Could you check a few things on this model? Use its own coordinates, in mm. Give positions to 0.01 mm unless a question says otherwise; leave off trailing zeros. Write each loop counter-clockwise with the first axis right and the second up, starting at its lowest first coordinate (ties: lowest second). Pieces come first, ordered by that corner, then holes. Notation, with made-up numbers: (9, 60.5) - (36, 60.5) arc R16 ccw to (36, 65.5) - close; hole circle Ø9 at (70.5, 75). An arc over 180 degrees is marked (long way). Write item = value, one per line.
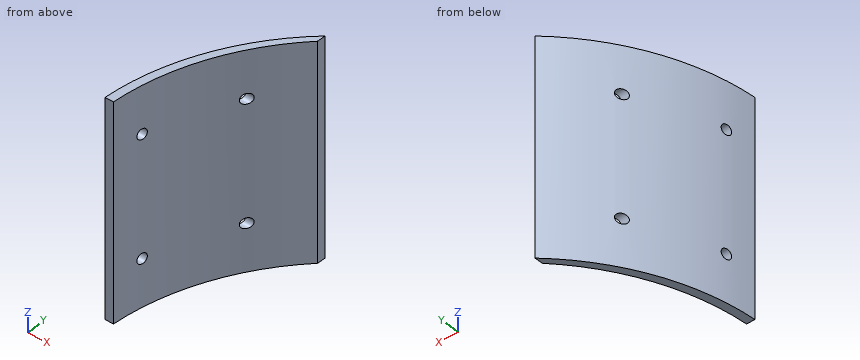
Autodesk Inventor part; units mm, degrees
ref_plane "YZ Plane" through (0, 0, 0) normal (1, 0, 0) x (0, 1, 0)
ref_plane "XZ Plane" through (0, 0, 0) normal (0, 1, 0) x (-1, 0, 0)
ref_plane "XY Plane" through (0, 0, 0) normal (0, 0, 1) x (1, 0, 0)
sketch "Sketch1" plane through (0, 0, 0) normal (0, 0, 1) x (1, 0, 0)
  arc A0 (45, 98) -> (0, 0) centre (139.9137, -4.9145) ccw
  line L0 (45, 98) -> (45, 93)
  line L1 (0, 0) -> (5, 0)
  arc A1 (45, 93) -> (5, 0) centre (144.908, -5.0734) ccw
  dimension "d0" = 140
  dimension "d1" = 98
  dimension "d3" = 45
  dimension "d4" = 5
  dimension "d5" = 5
  dimension "d6" = 140
extrude "Extrusion1" add sketch "Sketch1" along normal blind 125
sketch "Sketch2" plane through (0, 0, 0) normal (1, 0, 0) x (0, 1, 0)
  circle A0 centre (67.5, 27.5) radius 3
  circle A1 centre (17.5, 27.5) radius 3
  line L0 (98, 0) -> (98, 125)
  circle A2 centre (67.5, 97.5) radius 3
  circle A3 centre (17.5, 97.5) radius 3
  point P0 (0, 0)
  dimension "d9" = 6
  dimension "d10" = 6
  dimension "d11" = 27.5
  dimension "d12" = 50
  dimension "d13" = 30.5
  dimension "d14" = 6
  dimension "d15" = 6
  dimension "d16" = 70
extrude "Extrusion2" cut sketch "Sketch2" along normal through all
properties part number "SJ009" material "ABS Plastic"
1. If we section it at B-B, the plane z = 97.5: Please give me the cut outline in (x, y), and give its area (3 significant figures).
Filled sheet:
outline = (0, 0) - (5, 0) arc R140 cw to (6.28, 14.5) - (1.27, 14.5) arc R140 ccw to start; (2.24, 20.5) - (7.26, 20.5) arc R140 cw to (23.42, 64.5) - (18.33, 64.5) arc R140 ccw to start; (21.96, 70.5) - (27.06, 70.5) arc R140 cw to (45, 93) - (45, 98) arc R140 ccw to start
area = 423 mm2
2. If we section it at A-A, the plane y = 17: Please give me the cut outline in (x, z).
Filled sheet:
outline = (1.64, 0) - (6.66, 0) - (6.66, 24.54) - (1.64, 24.54) - close; (1.64, 30.46) - (6.66, 30.46) - (6.66, 94.54) - (1.64, 94.54) - close; (1.64, 100.46) - (6.66, 100.46) - (6.66, 125) - (1.64, 125) - close
3. I need wall thicknesses on line 1 (Z direction, x = 2.5, y = 17.5); line 2 (Y direction, x = 23, z = 97); line 3 (X direction, y = 12.5, z = 118). Which ranges of each line are inside material? Lowest first, please.
Filled sheet:
line_1 = 0 to 24.5, 30.5 to 94.5, 100.5 to 125
line_2 = 63.76 to 64.54, 70.46 to 72.1
line_3 = 1 to 6.02
4. For pin 1 (10 mm diameter, centred on x = 8.5, z = 51.5, fed in from +Y); pin 2 (1.5 mm diameter, centred on y = 76.5, z = 59.5, fed in from -X); pin 3 (7 mm diameter, centred on y = 17.5, z = 97.5, fed in from +X); pin 4 (5 mm diameter, centred on y = 17.5, z = 27.5, fed in from +X), each with a flat end and sliding along its axis, tell me the tip position at first contact or that it passes through.
Filled sheet:
pin_1 = 55.25
pin_2 = 25.49
pin_3 = 7.36
pin_4 = through
5. If we section it at C-C, the plane x = 12: Please give me the cut outline in (y, z).
Filled sheet:
outline = (38.92, 0) - (51.99, 0) - (51.99, 125) - (38.92, 125) - close
6. If we section it at D-D, the plane z = 65: Please give me the cut outline in (x, y).
Filled sheet:
outline = (0, 0) - (5, 0) arc R140 cw to (45, 93) - (45, 98) arc R140 ccw to start
